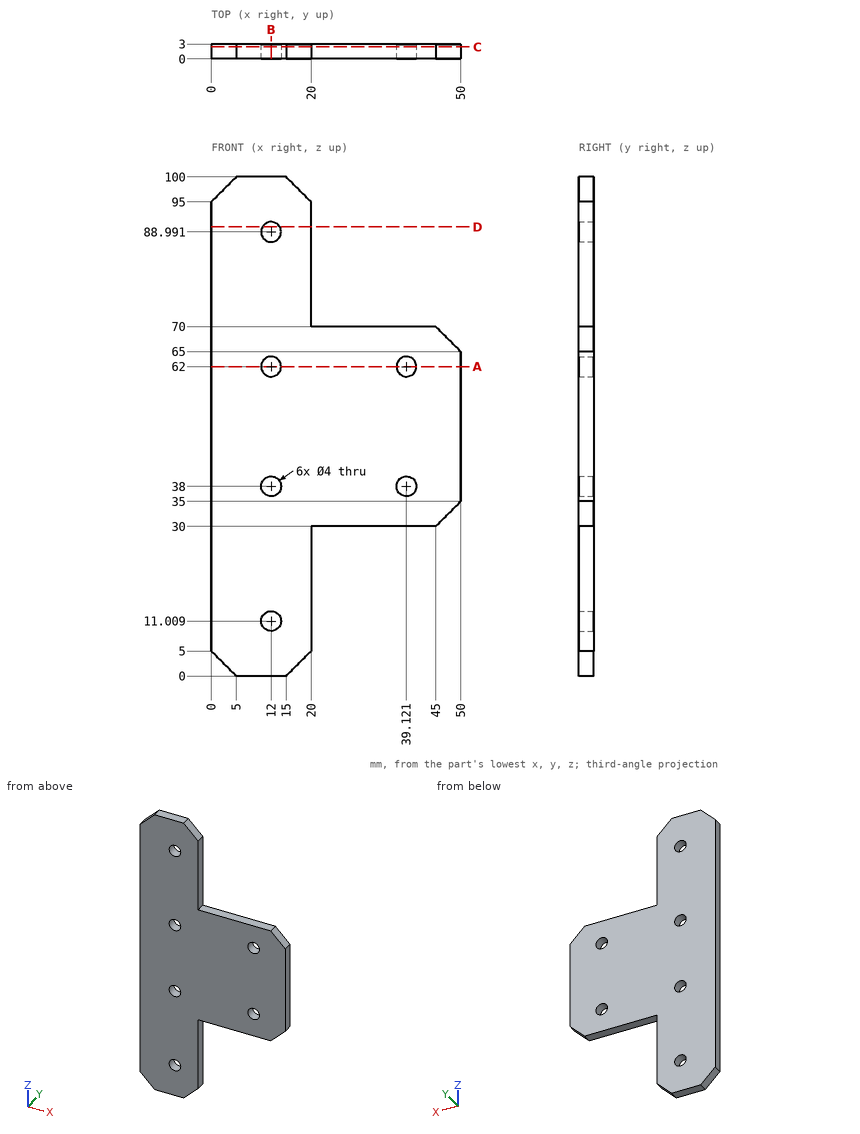
The drawing under review shows one solid part. Ordinate dimensions are in mm from its lowest x, y, z. Give positions to 0.01 mm unless a question says otherwise; leave off trailing zeros. Write each loop counter-clockwise with the first axis right and the second up, starting at its lowest first coordinate (ties: lowest second). Pieces come first, ordered by that corner, then holes. Notation, with made-up numbers: (-20.75, 31.5) - (28.25, 31.5) arc R22 ccw to (28.25, 63.5) - close; hole circle Ø9 at (40, -13). An arc over 180 degrees is marked (long way). Answer in a Markdown table with one row per item. Add a question column.
1. We need section D-D on z = 90. Write out the cut boundary in (x, y).
2. We need section C-C on y = 2.4. Write out the cut boundary in (x, z).
3. We need section A-A on z = 62. Write out the cut boundary in (x, y).
4. Insertion check: P1, Ø1, axis at x = 32, y = 1, coming from the -Z side; P2, Ø1, axis at x = 24, y = 2.5, coming from the +Z side; P3, Ø0.9, axis at y = 1.5, z = 16.5, coming from the +X side. Each pin has a flat end and moves straight along its axis. Give the tip position at first contact, or say it passes through.
5. We need section B-B on x = 12. Write out the cut boundary in (y, z), then the cut area to 3 significant figures.
6. Wall thickness on line 1 along Z through (x, y) = (12, 2.3); line 2 along X through (y, z) = (0.95, 11); line 3 along X through (y, z) = (1.85, 21): over which ranges is each line inside the solid? List them lowest first. Write a range as [from, to].
Ans:
| question | item | result |
|---|---|---|
| 1 | outline | (0, 0) - (10.27, 0) - (10.27, 3) - (0, 3) - close; (13.73, 0) - (20, 0) - (20, 3) - (13.73, 3) - close |
| 2 | outline | (0, 5) - (5, 0) - (15, 0) - (20, 5) - (20, 30) - (45, 30) - (50, 35) - (50, 65) - (45, 70) - (20, 70) - (20, 95) - (15, 100) - (5, 100) - (0, 95) - close; hole circle Ø4 at (12, 11.01); hole circle Ø4 at (12, 38); hole circle Ø4 at (12, 62); hole circle Ø4 at (12, 88.99); hole circle Ø4 at (39.12, 38); hole circle Ø4 at (39.12, 62) |
| 3 | outline | (0, 0) - (10, 0) - (10, 3) - (0, 3) - close; (14, 0) - (37.12, 0) - (37.12, 3) - (14, 3) - close; (41.12, 0) - (50, 0) - (50, 3) - (41.12, 3) - close |
| 4 | P1 | stops at z = 30 |
| 4 | P2 | stops at z = 70 |
| 4 | P3 | stops at x = 20 |
| 5 | outline | (0, 0) - (3, 0) - (3, 9.01) - (0, 9.01) - close; (0, 13.01) - (3, 13.01) - (3, 36) - (0, 36) - close; (0, 40) - (3, 40) - (3, 60) - (0, 60) - close; (0, 64) - (3, 64) - (3, 86.99) - (0, 86.99) - close; (0, 90.99) - (3, 90.99) - (3, 100) - (0, 100) - close |
| 5 | area | 252 mm^2 |
| 6 | line 1 | z = [0, 9.01], [13.01, 36], [40, 60], [64, 86.99], [90.99, 100] |
| 6 | line 2 | x = [0, 10], [14, 20] |
| 6 | line 3 | x = [0, 20] |
